Read the model definition and answer for the solid it produces. Units are mm, in the model's axes. Face numbers are marked on the shaded views. Round coordinates to 2 decimals unless told otherwise and drop trailing zeros. Order: outer loops, then holes, each group sorted by start corner. A loop starts at its lowest first (then second) coordinate and runs counter-clockwise, first axis right, second up. Notation, with made-up numbers: (22.25, 84.25) - (45.25, 84.25) arc R21 ccw to (45.25, 106.25) - close; hole circle Ø8 at (52, 35). An arc over 180 degrees is marked (long way). Answer as a JSON object with one key per item and string values. Group by question number.
Q1. Given pin 1 Ø6.5 at (x, y) = (-4, 29.5) entering from -Z; pin 2 Ø4 at (x, y) = (-4, 26.5) entering from +Z, each flat-ended and moving along its own axis, determine where each tip first touches the part or whether it passes through.
Q2. A cutting plane is placed at B-B on x = -5.5. Determine the outline of the cut face in (y, z).
Q3. The mould has two halves that part along Y. Classify the marked faces 1, 2, 3 and 4: pulls with the +Y half, pulls with the -Y half, needs draft (parallel to the pull), parting line crosses it, or undercut.
Q4. A cutting plane is placed at A-A on z = 3.75. Determine the outline of the cut face in (x, y), and give its area (3 significant figures).
Q5. Consider line 1 (Z direction, x = -2.5, y = 25); line 2 (Y direction, x = -7.5, z = 3.5); line 3 (Y direction, x = -5.25, z = -1.25). Determine where each line is inside the solid, lowest interval first.
Q6. A cutting plane is placed at C-C on y = -30. Determine the outline of the cut face in (x, z).
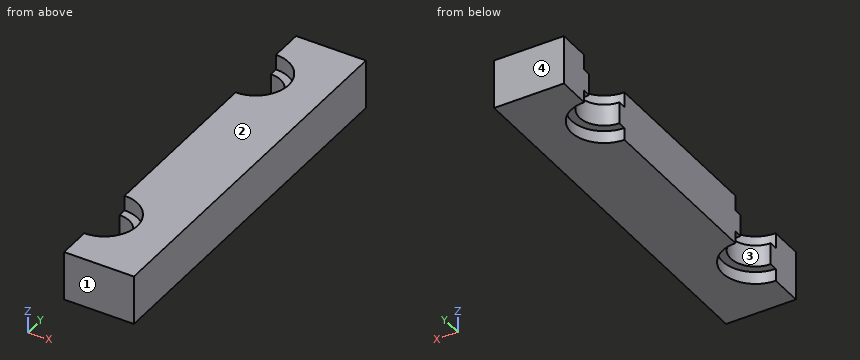
```python
from build123d import *

# Parameters (mm, degrees)
PAD_DEPTH       = 6
POCKET_DEPTH    = 3.7
POCKET001_DEPTH = 3


with BuildPart() as part:
    # Sketch → Pad (new body, symmetric)
    with BuildSketch(Plane.XY):
        with BuildLine():
            Line((-8.5, 36), (-8.5, 46))
            Line((-8.5, 46), (8.5, 46))
            Line((8.5, 46), (8.5, -46))
            Line((8.5, -46), (-8.500001, -46))
            Line((-8.500001, -46), (-8.500001, -36))
            ThreePointArc((-8.500001, -36), (-2.5, -30), (-8.5, -24))
            Line((-8.5, 24), (-8.5, -24))
            ThreePointArc((-8.5, 24), (-2.5, 30), (-8.5, 36))
        make_face()
    extrude(amount=PAD_DEPTH, both=True)

    # Sketch001 → Pocket (cut)
    with BuildSketch(Plane.XY.offset(6)):
        with BuildLine():
            ThreePointArc((-8.500034, -38), (-0.500033, -30.000017), (-8.5, -22))
            Line((-8.5, -22), (-18.5, -21.999958))
            Line((-18.5, -21.999958), (-18.5, -38))
            Line((-18.5, -38), (-8.500034, -38))
        make_face()
        with BuildLine():
            ThreePointArc((-8.5, 22), (-0.5, 30), (-8.5, 38))
            Line((-8.5, 38), (-18.5, 38))
            Line((-18.5, 38), (-18.5, 22))
            Line((-18.5, 22), (-8.5, 22))
        make_face()
    extrude(amount=-POCKET_DEPTH, mode=Mode.SUBTRACT)

    # Sketch002 → Pocket001 (cut)
    with BuildSketch(Plane(origin=(0, 0, -6), x_dir=(1, 0, 0), z_dir=(0, 0, -1))):
        with BuildLine():
            ThreePointArc((-8.5, 22), (-0.5, 30), (-8.5, 38))
            Line((-8.5, 38), (-24.5, 38))
            Line((-24.5, 38), (-24.5, 22))
            Line((-24.5, 22), (-8.5, 22))
        make_face()
        with BuildLine():
            ThreePointArc((-8.5, -38), (-0.5, -30), (-8.5, -22))
            Line((-8.5, -22), (-24.5, -22))
            Line((-24.5, -22), (-24.5, -38))
            Line((-24.5, -38), (-8.5, -38))
        make_face()
    extrude(amount=-POCKET001_DEPTH, mode=Mode.SUBTRACT)


solid = part.part
```
Result set:
{
 "1": {"pin 1": "stops at z = -3", "pin 2": "stops at z = 2.3"},
 "2": {"outline": "(-46, -6) - (-37.42, -6) - (-37.42, -3) - (-35.2, -3) - (-35.2, 2.3) - (-37.42, 2.3) - (-37.42, 6) - (-46, 6) - close; (-24.8, -3) - (-22.58, -3) - (-22.58, -6) - (22.58, -6) - (22.58, -3) - (24.8, -3) - (24.8, 2.3) - (22.58, 2.3) - (22.58, 6) - (-22.58, 6) - (-22.58, 2.3) - (-24.8, 2.3) - close; (35.2, -3) - (37.42, -3) - (37.42, -6) - (46, -6) - (46, 6) - (37.42, 6) - (37.42, 2.3) - (35.2, 2.3) - close"},
 "3": {"face 1": "pulls with the -Y half", "face 2": "needs draft", "face 3": "undercut", "face 4": "pulls with the +Y half"},
 "4": {"outline": "(-8.5, -46) - (8.5, -46) - (8.5, 46) - (-8.5, 46) - (-8.5, 38) arc R8 cw to (-8.5, 22) - (-8.5, -22) arc R8 cw to (-8.5, -38) - close", "area": "1,360 mm²"},
 "5": {"line 1": "z = -3 to 2.3", "line 2": "y = -46 to -37.94, -22.06 to 22.06, 37.94 to 46", "line 3": "y = -46 to -35.04, -24.96 to 24.96, 35.04 to 46"},
 "6": {"outline": "(-2.5, -3) - (-0.5, -3) - (-0.5, -6) - (8.5, -6) - (8.5, 6) - (-0.5, 6) - (-0.5, 2.3) - (-2.5, 2.3) - close"}
}
